Design review of the part built by this model. Coordinates are the model's own, in mm. A direction names the side the tool comes from. Coordinates: 2 decimals unless noted, no trailing zeros. Loops run counter-clockwise (first coordinate to the right, second up) from the corner with the lowest first, then second, coordinate; pieces in that order, holes last. Notation, with made-up numbers: (52, -12.75) - (99, -12.75) arc R5 ccw to (99, -5.75) - close; hole circle Ø3 at (29.5, -35.75). An arc over 180 degrees is marked (long way). Return JSON: item names as keys, results as strings. Group by question number.
from build123d import *

# Parameters (mm, degrees)
BOSS_EXTRUDE1_DEPTH = 6
SKETCH2_R           = 3.5
BOSS_EXTRUDE2_DEPTH = 2.5
SKETCH4_R           = 2.05
CUT_EXTRUDE1_DEPTH  = 12.427306478
FILLET1_R           = 0.5


with BuildPart() as part:
    # Sketch1 → Boss-Extrude1 (new body)
    with BuildSketch(Plane(origin=(0, 0, 0), x_dir=(1, 0, 0), z_dir=(0, 1, 0))):
        Polygon((-2.886751346, 5), (-5.773502692, 0), (-2.886751346, -5), (2.886751346, -5), (5.773502692, 0), (2.886751346, 5), align=None)
    extrude(amount=BOSS_EXTRUDE1_DEPTH)

    # Sketch2 → Boss-Extrude2 (add)
    with BuildSketch(Plane(origin=(0, 6, 0), x_dir=(1, 0, 0), z_dir=(0, 1, 0))):
        with Locations(Location((0, 0, 0), (0, 0, 270))):
            Circle(SKETCH2_R)
    extrude(amount=BOSS_EXTRUDE2_DEPTH)

    # Sketch4 → Cut-Extrude1 (cut, through all)
    with BuildSketch(Plane(origin=(0, 8.5, 0), x_dir=(1, 0, 0), z_dir=(0, 1, 0))):
        with Locations(Location((1, 0, 0), (0, 0, 270))):
            Circle(SKETCH4_R)
    extrude(amount=-CUT_EXTRUDE1_DEPTH, mode=Mode.SUBTRACT)

    # Fillet1
    fillet1_edges = [part.edges().sort_by_distance(p)[0] for p in [
        (-4.330127019, 6, 2.5),
        (2.886751346, 3, -5),
        (5.773502692, 3, 0),
        (2.886751346, 3, 5),
        (-2.886751346, 3, 5),
        (-5.773502692, 3, 0),
        (-2.886751346, 3, -5),
        (0, 6, 5),
        (4.330127019, 6, 2.5),
        (4.330127019, 6, -2.5),
        (0, 6, -5),
        (4.330127019, 0, -2.5),
        (4.330127019, 0, 2.5),
        (0, 0, 5),
        (-4.330127019, 6, -2.5),
        (-4.330127019, 0, 2.5),
        (-4.330127019, 0, -2.5),
        (0, 0, -5),
    ]]
    fillet(fillet1_edges, radius=FILLET1_R)


solid = part.part
Item 1: Add section A-A (y = 0.75). State the section outline as (x, z) points, then the cut area to 3 significant figures.
Item 2: For P1, Ø4, axis at y = 3, z = -2, coming from the -X side; P2, Ø1.5, axis at y = 2, z = -2, coming from the +X side; P3, Ø1.5, axis at y = 6, z = 1.5, coming from the +X side, all flat-tipped, find the tip position at first contact; note any pin that passes through.
Item 3: Add section B-B (x = 0.5). State the section outline as (y, z) points.
Item 4: For faces 5 (the face through (-4.22, 5.85, -2.4)), 6 (the face through (1.5, 6, -3.4)), list the 3-axis set-ups (+Z, -Z, +X, -X, +Y, -Y) from which the entire face can be reached by the end or side of a thin tool; tool diameter is ignored.
Item 5: Add section C-C (y = 8). State the section outline as (x, z) points.
Item 6: To check wall thickness, follow line 1 (X direction, y = 4.75, z = 0); line 2 (Y direction, x = 3.5, z = 2.5); line 3 (Z direction, x = -0.25, y = 3). State the ranges of each line that lie inside material, in increasing order. Write a range as from..to.
Item 7: Draft analysis for pull direction Z (two halves, no side actions). For faces 1 (the face through (4.348, 2.965, -2.469)), 2 (the face through (4.22, 0.14, 2.39)), 3 (the face through (0.21, 4.31, 1.89)), 4 (the face through (-2, 8.5, 0)), state which applies: pulls with the +Z half, pulls with the -Z half, needs draft (parallel to the pull), parting line crosses it, or undercut.
Answers below:
{
 "1": {"outline": "(-5.63, -0.25) - (-3.03, -4.75) arc R0.5 ccw to (-2.6, -5) - (2.6, -5) arc R0.5 ccw to (3.03, -4.75) - (5.63, -0.25) arc R0.5 ccw to (5.63, 0.25) - (3.03, 4.75) arc R0.5 ccw to (2.6, 5) - (-2.6, 5) arc R0.5 ccw to (-3.03, 4.75) - (-5.63, 0.25) arc R0.5 ccw to start; hole circle Ø4.1 at (1, 0)", "area": "73.3 mm^2"},
 "2": {"P1": "stops at x = -5.7", "P2": "stops at x = 5.05", "P3": "stops at x = 5.26"},
 "3": {"outline": "(0, -4.5) arc R0.5 ccw to (0.5, -5) - (5.5, -5) arc R0.5 ccw to (6, -4.5) - (6, -3.46) - (8.5, -3.46) - (8.5, -1.99) - (0, -1.99) - close; (0, 1.99) - (8.5, 1.99) - (8.5, 3.46) - (6, 3.46) - (6, 4.5) arc R0.5 ccw to (5.5, 5) - (0.5, 5) arc R0.5 ccw to (0, 4.5) - close"},
 "4": {"face 5": "-Z, -X, +Y", "face 6": "+Y"},
 "5": {"outline": "circle Ø7 at (0, 0); hole circle Ø4.1 at (1, 0)"},
 "6": {"line 1": "x = -5.7..-1.05, 3.05..5.7", "line 2": "y = 0..6", "line 3": "z = -5..-1.62, 1.62..5"},
 "7": {"face 1": "pulls with the -Z half", "face 2": "pulls with the +Z half", "face 3": "undercut", "face 4": "needs draft"}
}
